Can you work these out from the model? Positions are in its coordinate system, mm. A direction names the side the tool comes from. Coordinates: 2 decimals unless noted, no trailing zeros. Loops run counter-clockwise (first coordinate to the right, second up) from the corner with the lowest first, then second, coordinate; pieces in that order, holes last. Notation, with made-up numbers: M 88.5,9 L 130.5,9 A22 cw 130.5,21 Z; hole C -11.5,65.5 d8. An arc over 180 degrees is marked long. Return JSON: item names as keys, results as strings. Group by question number.
```python
from build123d import *


with BuildPart() as part:
    # Skizze1 → Rotation1 (revolve)
    with BuildSketch(Plane.XY, mode=Mode.PRIVATE) as rotation1_sk:
        Polygon((168.152402442, 0), (168.152402442, 26.5), (169.152402442, 27.5), (184.152402442, 27.5), (212.152402442, 27.5), (212.152402442, 29), (213.152402442, 30), (267.152402442, 30), (267.152402442, 32.5), (273.152402442, 32.5), (273.152402442, 30), (285.152402442, 30), (285.152402442, 27.5), (297.652402442, 27.5), (316.152402442, 27.5), (317.152402442, 26.5), (317.152402442, 25), (331.652402442, 25), (334.152402442, 23.556624327), (334.152402442, 20), (393.152402442, 20), (394.152402442, 19), (394.152402442, 0), align=None)
    revolve(rotation1_sk.sketch.rotate(Axis((168.152402442, 0, 0), (1, 0, 0)), 90), axis=Axis((168.152402442, 0, 0), (1, 0, 0)))  # turned: the seam where the file's is


solid = part.part
```
1) Suppose I cut it at A-A, the plane x = 248. List the corners of the cut face in (y, z) for me.
2) If I drill on line 1 (X direction, y = 27.5, z = -14.5); line 2 (X direction, y = -4.5, z = 25); line 3 (Y direction, x = 179, z = -16), over which ranges is the centre line in solid material (lowest first)? Write a range as from..to.
3) For faces 1 (the face through (300.435, 24.397, 12.69)), 2 (the face through (240.53, -25.296, 16.128)), 3 (the face through (168.152, 0, 0)), which set-ups out of +Z, -Z, +X, -X, +Y, -Y let a thin tool reach every point of the face, with its end or its side?
4) For pin 1 (2 mm diameter, centred on x = 344, z = -13, fed in from +Y); pin 2 (3 mm diameter, centred on x = 280.5, z = 16, fed in from -Y); pin 3 (1.5 mm diameter, centred on x = 202.5, y = 5.5, fed in from +Z), each with a flat end and sliding along its axis, tell me the tip position at first contact or that it passes through.
5) Suppose I cut it at B-B, the plane x = 301.5. List the corners of the cut face in (y, z) for me, then the cut area to 3 significant figures.
Returned:
{
 "1": {"outline": "C 0,0 d60"},
 "2": {"line 1": "x = 267.15..273.15", "line 2": "x = 168.15..317.15", "line 3": "y = -22.37..22.37"},
 "3": {"face 1": "+X", "face 2": "-X", "face 3": "+Z, -Z, -X, +Y, -Y"},
 "4": {"pin 1": "stops at y = 16", "pin 2": "stops at y = -26.26", "pin 3": "stops at z = 27.09"},
 "5": {"outline": "C 0,0 d55", "area": "2,380 mm²"}
}
